Can you work these out from the drawing? Everything is in mm from the part's minimum corner. Give positions to 0.01 mm unless a question says otherwise; leave off trailing zeros. Order: outer loops, then holes, each group sorted by start corner. A loop starts at its lowest first (then second) coordinate and runs counter-clockwise, first axis right, second up. Notation, with made-up numbers: (52.5, 39.25) -> (103.5, 39.25) arc R21 cw to (103.5, 75.25) -> close; hole circle Ø7 at (82, 19). An arc over 180 degrees is marked (long way). One line per item, written item: value.
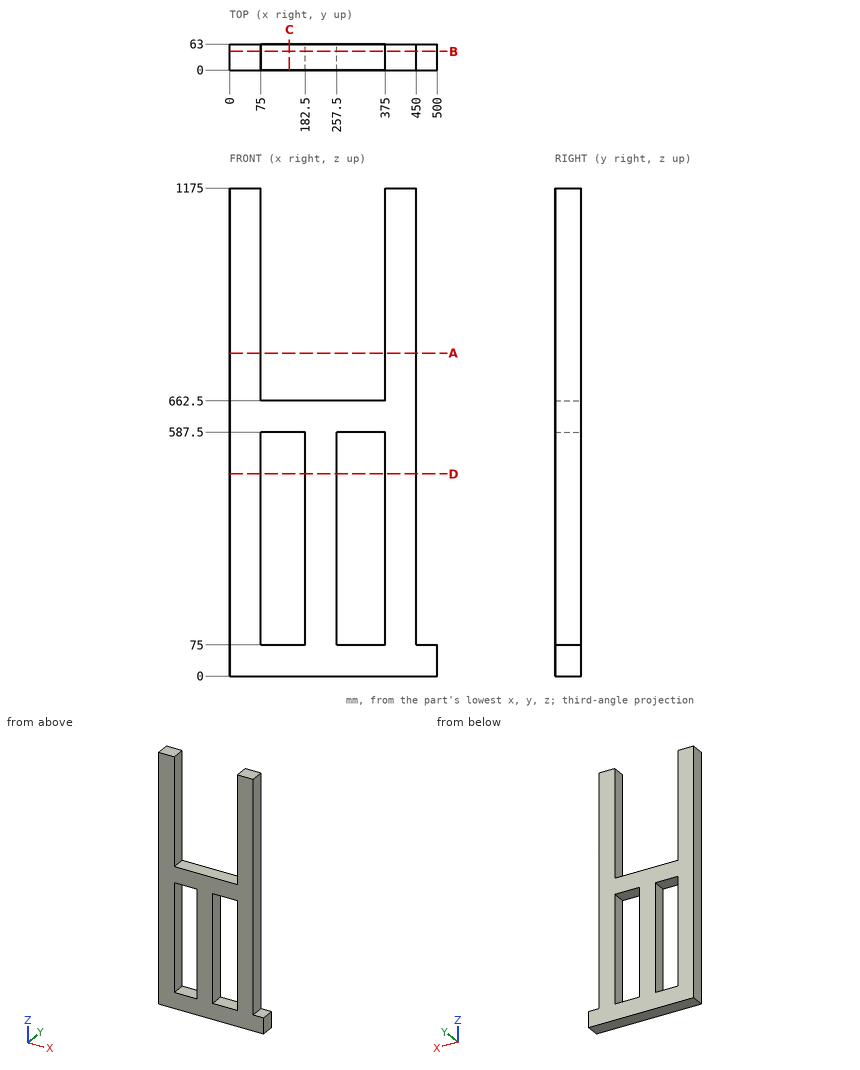
1) For P1, Ø19, axis at y = 45, z = 206.5, coming from the +X side; P2, Ø6, axis at x = 215.5, y = 24, coming from the +Z side, each with a flat end and sliding along its axis, tell me the tip position at first contact or that it passes through.
Answer below:
P1: stops at x = 450
P2: stops at z = 662.5
2) Suppose I cut it at B-B, the plane y = 45. Write out the boundary of the cut face in (x, z).
Answer below:
outline: (0, 0) -> (500, 0) -> (500, 75) -> (450, 75) -> (450, 1175) -> (375, 1175) -> (375, 662.5) -> (75, 662.5) -> (75, 1175) -> (0, 1175) -> close; hole (75, 75) -> (182.5, 75) -> (182.5, 587.5) -> (75, 587.5) -> close; hole (257.5, 75) -> (375, 75) -> (375, 587.5) -> (257.5, 587.5) -> close
3) Suppose I cut it at D-D, the plane z = 487. Write out the boundary of the cut face in (x, y).
Answer below:
outline: (0, 0) -> (75, 0) -> (75, 63) -> (0, 63) -> close; (182.5, 0) -> (257.5, 0) -> (257.5, 63) -> (182.5, 63) -> close; (375, 0) -> (450, 0) -> (450, 63) -> (375, 63) -> close
4) Suppose I cut it at A-A, the plane z = 777.5. Write out the boundary of the cut face in (x, y).
Answer below:
outline: (0, 0) -> (75, 0) -> (75, 63) -> (0, 63) -> close; (375, 0) -> (450, 0) -> (450, 63) -> (375, 63) -> close
5) If I drill on line 1 along X through (y, z) = (43, 485); line 2 along Z through (x, y) = (131.5, 52); line 3 along X through (y, z) = (13, 1116), over which ranges is the centre line in solid material (lowest first)?
Answer below:
line 1: x = 0 to 75, 182.5 to 257.5, 375 to 450
line 2: z = 0 to 75, 587.5 to 662.5
line 3: x = 0 to 75, 375 to 450
6) Suppose I cut it at C-C, the plane x = 144. Write out the boundary of the cut face in (y, z), then the cut area to 3 significant figures.
Answer below:
outline: (0, 0) -> (63, 0) -> (63, 75) -> (0, 75) -> close; (0, 587.5) -> (63, 587.5) -> (63, 662.5) -> (0, 662.5) -> close
area: 9,450 mm2
